```python
from build123d import *

# Parameters (mm, degrees)
BOX_SKETCH_W       = 80
BOX_SKETCH_H       = 80
BOX_EXTRUDE_DEPTH  = 80
BOX_FILLET_R       = 10
POLE_SKETCH_R      = 20
POLE_EXTRUDE_DEPTH = 100
HOLE_SKETCH_R      = 10
HOLE_CUT_DEPTH     = 80


with BuildPart() as part:
    # Box Sketch → Box Extrude (new body)
    with BuildSketch(Plane.XY):
        Rectangle(BOX_SKETCH_W, BOX_SKETCH_H)
    extrude(amount=BOX_EXTRUDE_DEPTH)

    # Box Fillet
    box_fillet_edges = [part.edges().sort_by_distance(p)[0] for p in [
        (-40, 0, 80),
        (0, -40, 80),
        (40, 0, 80),
        (0, -40, 0),
        (-40, 0, 0),
        (0, 40, 0),
        (40, 0, 0),
        (0, 40, 80),
        (40, -40, 40),
        (-40, -40, 40),
        (-40, 40, 40),
        (40, 40, 40),
    ]]
    fillet(box_fillet_edges, radius=BOX_FILLET_R)

    # Pole Sketch → Pole Extrude (add)
    with BuildSketch(Plane(origin=(0, 0, 0), x_dir=(-1, 0, 0), z_dir=(0, 0, -1))):
        with Locations(Location((0, 0, 0), (0, 0, 180))):
            Circle(POLE_SKETCH_R)
    extrude(amount=POLE_EXTRUDE_DEPTH)

    # Hole Sketch → Hole Cut (cut)
    with BuildSketch(Plane.ZY.offset(40)):
        with Locations(Location((40, 0, 0), (0, 0, 270))):
            Circle(HOLE_SKETCH_R)
    extrude(amount=-HOLE_CUT_DEPTH, mode=Mode.SUBTRACT)


solid = part.part
```
Can you work these out from the model? Positions are in its coordinate system, mm. A direction names the side the tool comes from. Coordinates: 2 decimals unless noted, no trailing zeros. Write each loop counter-clockwise with the first axis right and the second up, starting at its lowest first coordinate (ties: lowest second). Pieces come first, ordered by that corner, then holes. Notation, with made-up numbers: M 68,27.5 L 102,27.5 A18 ccw 102,32.5 Z; hole C 6.5,-20 d10. An arc over 180 degrees is marked long. Write item = value, one per line. Start each with the question number.
Q1. On a 3-axis mill with a long thin cutter (end or side, diameter ignored), from which of +Z, -Z, +X, -X, +Y, -Y can I reach the whole of each face in a straight line? I mean faces 4 (the face through (-0.4, 20.4, 0)), 5 (the face through (0, 40, 40)). Say none if no direction works.
Q2. If we section it at B-B, the plane y = 0: Write out the boundary of the cut face in (x, z).
Q3. If we section it at C-C, the plane z = 40: Write out the boundary of the cut face in (x, y).
Q4. If we section it at D-D, the plane y = 12: Write out the boundary of the cut face in (x, z), then the cut area to 3 significant figures.
Q5. If we section it at A-A, the plane x = 0: Write out the boundary of the cut face in (y, z), then the cut area to 3 significant figures.
Q6. Thinking about a two-plate mould opening in Z: for faces 1 (the face through (-37.15, 0.42, 3.01)), 2 (the face through (0, 0, 80)), 3 (the face through (-0.56, 2.17, 30.24)), which applies, released by +Z, released by -Z, zero draft, split by the parting line, or undercut?
Q7. I'm going to push flat-ended pins straight in: pin 1 (4 mm diameter, centred on x = -23, y = -11.5, fed in from -Z); pin 2 (2 mm diameter, centred on x = -10, z = -26, fed in from +Y); pin 3 (12 mm diameter, centred on x = 27.5, z = 1, fed in from -Y). Where does each tip first touch, or does it pass through?
Q8. If I drill on L1, parallel to Z at x = -2.5, y = 0; L2, parallel to Z at x = 28, y = 21.5; L3, parallel to Y at x = -25, z = 44.5, over which ranges is the centre line in solid material (lowest first)? Write a range as [from, to].
Check sheet entries:
q1.face_4 = -Z
q1.face_5 = +Z, -Z, +X, -X, +Y
q2.outline = M -40,10 A10 ccw -30,0 L -20,0 L -20,-100 L 20,-100 L 20,0 L 30,0 A10 ccw 40,10 L 40,30 L -40,30 Z; M -40,50 L 40,50 L 40,70 A10 ccw 30,80 L -30,80 A10 ccw -40,70 Z
q3.outline = M -40,-30 A10 ccw -30,-40 L 30,-40 A10 ccw 40,-30 L 40,-10 L -40,-10 Z; M -40,10 L 40,10 L 40,30 A10 ccw 30,40 L -30,40 A10 ccw -40,30 Z
q4.outline = M -40,10 A10 ccw -30,0 L -16,0 L -16,-100 L 16,-100 L 16,0 L 30,0 A10 ccw 40,10 L 40,70 A10 ccw 30,80 L -30,80 A10 ccw -40,70 Z
q4.area = 9,510 mm²
q5.outline = M -40,10 A10 ccw -30,0 L -20,0 L -20,-100 L 20,-100 L 20,0 L 30,0 A10 ccw 40,10 L 40,70 A10 ccw 30,80 L -30,80 A10 ccw -40,70 Z; hole C 0,40 d20
q5.area = 10,000 mm²
q6.face_1 = released by -Z
q6.face_2 = released by +Z
q6.face_3 = undercut
q7.pin_1 = 0
q7.pin_2 = 17.86
q7.pin_3 = -39.54
q8.L1 = [-100, 30], [50, 80]
q8.L2 = [0, 80]
q8.L3 = [-40, -8.93], [8.93, 40]
